Geometry: see drawing. Coordinates: mm, zero at the bounding-box minimum. A direction names the side the tool comes from. Round coordinates to 2 decimals unless told otherwise and drop trailing zeros. Write each loop counter-clockwise with the first axis right and the second up, starting at its lowest first coordinate (ties: lowest second). Pieces come first, ordered by that corner, then holes. Notation, with made-up numbers: M 61,35.25 L 70,35.25 A26 cw 70,57.25 Z; hole C -21,86.25 d4. An arc over 180 degrees is marked long. Use a Markdown table: item, result.
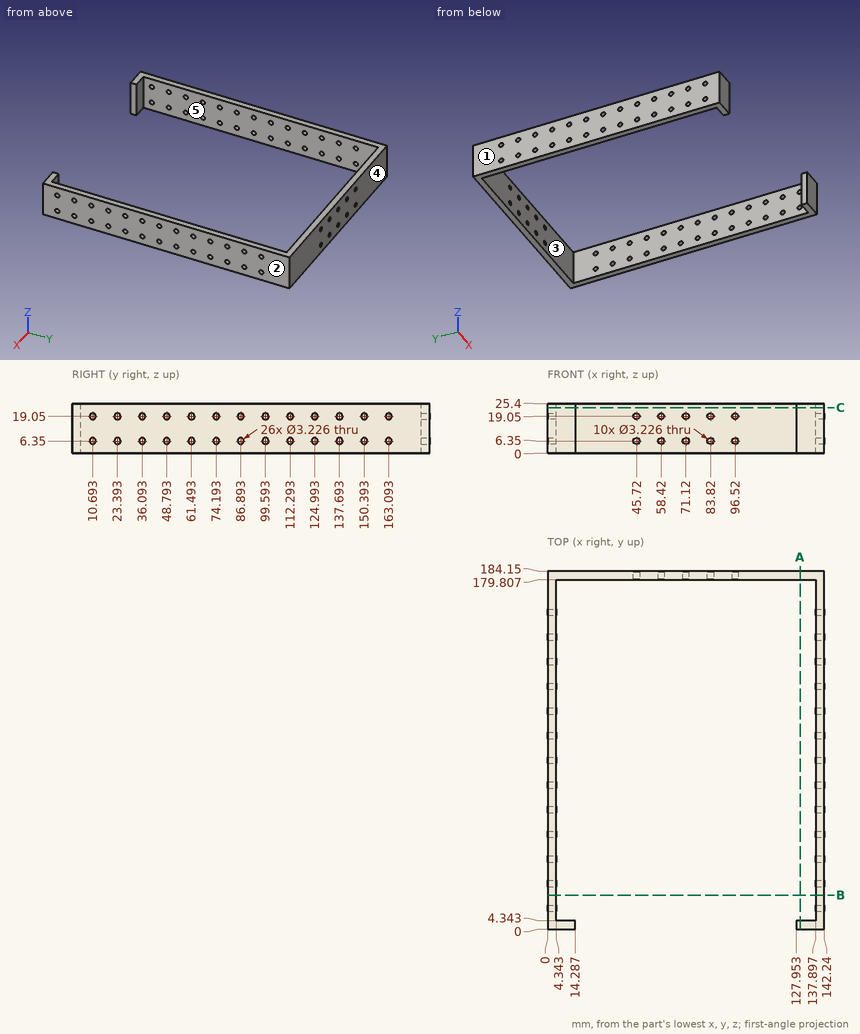
Q1. Reachability of the marked faces 4 and 5 from +Z, -Z, +X, -X, +Y, -Y: full face, straight path, thin tool, end or side. Return the list, or none.
Results are:
| item | result |
|---|---|
| face 4 | +Z, -Z, +X, -X, +Y |
| face 5 | +Z, -Z |
Q2. Mould query, pull axis X, two halves, no side actions, for the marked faces 1, 2 and 3. Classes: +X half, -X half, draft (parallel to the pull), parting line (faces both ways), or undercut.
Results are:
| item | result |
|---|---|
| face 1 | -X half |
| face 2 | +X half |
| face 3 | undercut |
Q3. Section C-C on z = 23.5. Return loops of the section in (x, y).
Results are:
| item | result |
|---|---|
| outline | M 0,0 L 14.29,0 L 14.29,4.34 L 4.34,4.34 L 4.34,179.81 L 137.9,179.81 L 137.9,4.34 L 127.95,4.34 L 127.95,0 L 142.24,0 L 142.24,184.15 L 0,184.15 Z |
Q4. Section B-B on y = 17.5. Return loops of the section in (x, z).
Results are:
| item | result |
|---|---|
| outline | M 0,0 L 4.34,0 L 4.34,25.4 L 0,25.4 Z; M 137.9,0 L 142.24,0 L 142.24,25.4 L 137.9,25.4 Z |
Q5. Section A-A on x = 130. Return loops of the section in (y, z).
Results are:
| item | result |
|---|---|
| outline | M 0,0 L 4.34,0 L 4.34,25.4 L 0,25.4 Z; M 179.81,0 L 184.15,0 L 184.15,25.4 L 179.81,25.4 Z |
Q6. Line query: L1, parallel to Z at x = 58.42, y = 181.95; L2, parallel to X at y = 165.5, z = 2.25; L3, parallel to Y at x = 100, z = 18.75. Output: solid intervals per line, ascending.
Results are:
| item | result |
|---|---|
| L1 | 0 to 4.74, 7.96 to 17.44, 20.66 to 25.4 |
| L2 | 0 to 4.34, 137.9 to 142.24 |
| L3 | 179.81 to 184.15 |
Q7. First-contact query: pin 1 Ø3.5 at (y, z) = (124.99, 19.05) entering from -X; pin 2 Ø1.9 at (y, z) = (36.09, 19.05) entering from -X; pin 3 Ø8 at (x, z) = (52.5, 11) entering from -Y. Flat tips, straight axial feed; report the tip coordinate or a pass-through.
Results are:
| item | result |
|---|---|
| pin 1 | x = 0 |
| pin 2 | through |
| pin 3 | y = 179.81 |
